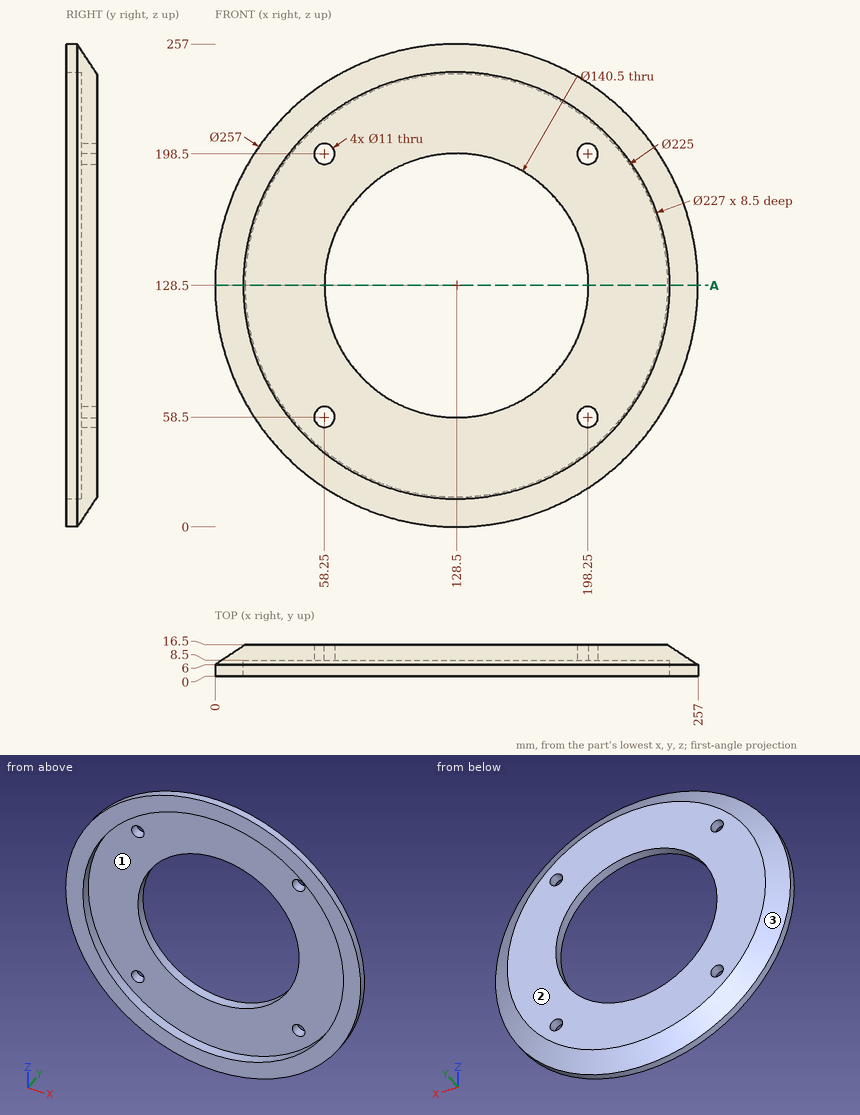
The drawing under review shows one solid part. Ordinate dimensions are in mm from its lowest x, y, z. Coordinates: 2 decimals unless noted, no trailing zeros. Order: outer loops, then holes, each group sorted by start corner. A loop starts at its lowest first (then second) coordinate and runs counter-clockwise, first axis right, second up. Notation, with made-up numbers: (76.5, 14.25) -> (128.5, 14.25) arc R14 ccw to (128.5, 32.25) -> close; hole circle Ø6 at (76, -21). An arc over 180 degrees is marked (long way). Answer in a Markdown table with one row per item. Add a question column.
Item 1: Clearance check with flat-ended pins moving along their axes: pin 1 (1 mm diameter, centred on y = 11.5, z = 141, fed in from -X); pin 2 (17.5 mm diameter, centred on x = 198.25, z = 58.5, fed in from -Y); pin 3 (1.5 mm diameter, centred on y = 6, z = 127.5, fed in from +X). State where each tip first meets the part, or that it passes through.
Item 2: We need section A-A on z = 128.5. Write out the cut boundary in (x, y), plus the area to 3 significant figures.
Item 3: To check wall thickness, follow probe 1 along Z at (x, y) = (128.5, 3.5); probe 2 along Y at (x, z) = (89, 187). State the ranges of each line that lie inside material, in increasing order.
Item 4: Mouldability with a two-part tool opening along Z and no side actions: class the marked faces 1, 2 and 3 as +Z half, -Z half, draft (parallel to the pull), parting line (faces both ways), or undercut.
Final values:
| question | item | result |
|---|---|---|
| 1 | pin 1 | stops at x = 8.27 |
| 1 | pin 2 | stops at y = 8.5 |
| 1 | pin 3 | stops at x = 257 |
| 2 | outline | (0, 0) -> (15, 0) -> (15, 8.5) -> (58.25, 8.5) -> (58.25, 16.5) -> (16, 16.5) -> (0, 6) -> close; (198.75, 8.5) -> (242, 8.5) -> (242, 0) -> (257, 0) -> (257, 6) -> (241, 16.5) -> (198.75, 16.5) -> close |
| 2 | area | 1,020 mm2 |
| 3 | probe 1 | z = 0 to 15, 242 to 257 |
| 3 | probe 2 | y = 8.5 to 16.5 |
| 4 | face 1 | undercut |
| 4 | face 2 | draft |
| 4 | face 3 | parting line |
